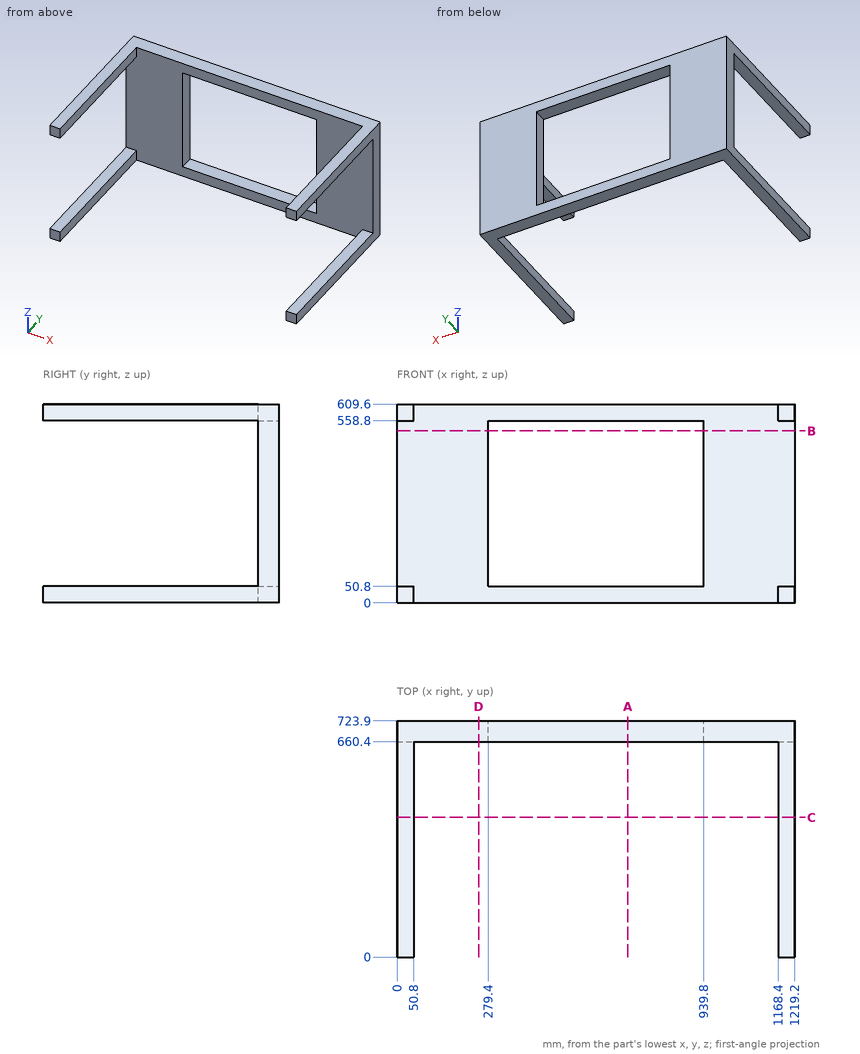
Geometry check sheet. Reference: drawing and pictorial views, mm from the part's lowest x, y, z. Round coordinates to 2 decimals unless told otherwise and drop trailing zeros. Loops run counter-clockwise (first coordinate to the right, second up) from the corner with the lowest first, then second, coordinate; pieces in that order, holes last. Notation, with made-up numbers: (-38, 21) -> (-32, 21) arc R13 ccw to (-32, 27) -> close; hole circle Ø2 at (-9.75, 89). An arc over 180 degrees is marked (long way). Answer as a JSON object with one key per item and string values.
Q1. Section check D-D (x = 249.5). Record the boundary of the cut face in (y, z), then the cut area to 3 significant figures.
Data:
{"outline": "(660.4, 0) -> (723.9, 0) -> (723.9, 609.6) -> (660.4, 609.6) -> close", "area": "38,700 mm2"}
Q2. Go/stop test with a flat-tipped pin: P1, Ø3, axis at x = 997, z = 476, coming from the -Y side. Record where the tip stops, or that it passes through.
Data:
{"P1": "stops at y = 660.4"}
Q3. Section check B-B (z = 527). Record the boundary of the cut face in (x, y).
Data:
{"outline": "(0, 660.4) -> (279.4, 660.4) -> (279.4, 723.9) -> (0, 723.9) -> close; (939.8, 660.4) -> (1219.2, 660.4) -> (1219.2, 723.9) -> (939.8, 723.9) -> close"}
Q4. Section check C-C (y = 428.5). Record the boundary of the cut face in (x, z), then the cut area to 3 significant figures.
Data:
{"outline": "(0, 0) -> (50.8, 0) -> (50.8, 50.8) -> (0, 50.8) -> close; (0, 558.8) -> (50.8, 558.8) -> (50.8, 609.6) -> (0, 609.6) -> close; (1168.4, 0) -> (1219.2, 0) -> (1219.2, 50.8) -> (1168.4, 50.8) -> close; (1168.4, 558.8) -> (1219.2, 558.8) -> (1219.2, 609.6) -> (1168.4, 609.6) -> close", "area": "10,300 mm2"}
Q5. Section check A-A (x = 707). Record the boundary of the cut face in (y, z), then the cut area to 3 significant figures.
Data:
{"outline": "(660.4, 0) -> (723.9, 0) -> (723.9, 50.8) -> (660.4, 50.8) -> close; (660.4, 558.8) -> (723.9, 558.8) -> (723.9, 609.6) -> (660.4, 609.6) -> close", "area": "6,450 mm2"}
Q6. Scan lines: line 1 (X direction, y = 190, z = 582); line 2 (Y direction, x = 204, z = 422). Record each from-to range of solid material in increasing order. Write a range as from..to.
Data:
{"line 1": "x = 0..50.8, 1168.4..1219.2", "line 2": "y = 660.4..723.9"}
